Design review of the part built by this model. Coordinates are the model's own, in mm. Face numbers are marked on the shaded views. Round coordinates to 2 decimals unless told otherwise and drop trailing zeros. Write each loop counter-clockwise with the first axis right and the second up, starting at its lowest first coordinate (ties: lowest second). Pieces come first, ordered by that corner, then holes. Notation, with made-up numbers: (65.5, -26.75) - (89.5, -26.75) arc R21 ccw to (89.5, 2.25) - close; hole circle Ø2 at (-31, 34.5). An arc over 180 degrees is marked (long way). Use one line per item in the form item = value.
```python
from build123d import *

# Parameters (mm, degrees)
F0_W     = 50.6464093924
F0_H     = 100.5250141025
F1_DEPTH = 0.254
F0_W_2   = 58.674
F0_H_2   = 123.952
F2_DEPTH = 7.874
F3_R     = 9.8113639175
F4_R     = 9.8044
F6_W     = 12.2285038233
F6_H     = 3.6733425222
F7_DEPTH = 17.272
F8_R     = 2.2102361545
F9_DEPTH = 12.192


# Not quite as in the source:
# - the program builds the solid bodies; features that only make, move or delete a surface that nothing else refers to are left out


with BuildPart() as f1:
    # F0 (on Top) → F1 (new body)
    with BuildSketch(Plane.XY):
        with Locations((55.8215677738, 54.941402014)):
            Rectangle(F0_W, F0_H)
    extrude(amount=F1_DEPTH)

    # F0 (on Top) → F2 (join)
    with BuildSketch(Plane.XY):
        with Locations((55.8215677738, 54.941402014)):
            Rectangle(F0_W_2, F0_H_2)
        with Locations((55.8215677738, 54.941402014)):
            Rectangle(F0_W, F0_H, mode=Mode.SUBTRACT)
    extrude(amount=F2_DEPTH)

    # F3
    f3_edges = [f1.edges().sort_by_distance(p)[0] for p in [
        (26.484568, 116.917402, 3.937),
    ]]
    fillet(f3_edges, radius=F3_R)

    # F4
    f4_edges = [f1.edges().sort_by_distance(p)[0] for p in [
        (85.158568, 116.917402, 3.937),
    ]]
    fillet(f4_edges, radius=F4_R)

    # F6 (on face) → F7 (cut)
    with BuildSketch(Plane.XZ.offset(7.034597986)):
        with Locations((55.8215677738, 4.2473026551)):
            Rectangle(F6_W, F6_H)
    extrude(amount=-F7_DEPTH, mode=Mode.SUBTRACT)

    # F8 (on face) → F9 (cut)
    with BuildSketch(Plane.XZ.offset(7.034597986)):
        with Locations((35.0567772985, 3.8737377618)):
            Circle(F8_R)
    extrude(amount=-F9_DEPTH, mode=Mode.SUBTRACT)


solid = f1.part
```
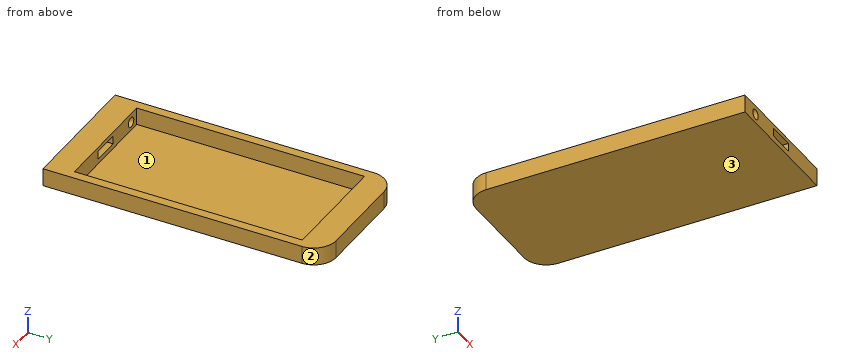
Q1. We need section D-D on x = 35. Write out the cut boundary in (y, z).
Calculated:
outline = (-7.03, 0) - (116.83, 0) - (116.83, 7.87) - (105.2, 7.87) - (105.2, 0.25) - (4.68, 0.25) - (4.68, 1.66) - (-7.03, 1.66) - close; (-7.03, 6.08) - (4.68, 6.08) - (4.68, 7.87) - (-7.03, 7.87) - close
Q2. We need section B-B on y = 6.5. Write out the cut boundary in (x, z).
Calculated:
outline = (26.48, 0) - (85.16, 0) - (85.16, 7.87) - (81.14, 7.87) - (81.14, 0.25) - (30.5, 0.25) - (30.5, 7.87) - (26.48, 7.87) - close
Q3. We need section A-A on x = 53.5. Write out the cut boundary in (y, z).
Calculated:
outline = (-7.03, 0) - (116.92, 0) - (116.92, 7.87) - (105.2, 7.87) - (105.2, 0.25) - (4.68, 0.25) - (4.68, 2.41) - (-7.03, 2.41) - close; (-7.03, 6.08) - (4.68, 6.08) - (4.68, 7.87) - (-7.03, 7.87) - close
Q4. To check wall thickness, follow line 1 along Y through (x, z) = (43, 7); line 2 along X through (y, z) = (61.5, 5.25); line 3 along Z through (x, y) = (61, 79). State the ranges of each line that lie inside material, in increasing order. Write a range as from..to.
Calculated:
line_1 = -7.03..4.68, 105.2..116.92
line_2 = 26.48..30.5, 81.14..85.16
line_3 = 0..0.25
Q5. For P1, Ø6, axis at x = 67, y = 75, coming from the +Z side, flat-tipped, find the tip position at first contact; note if it passes through.
Calculated:
P1 = 0.25
Q6. We need section C-C on x = 46. Write out the cut boundary in (y, z).
Calculated:
outline = (-7.03, 0) - (116.92, 0) - (116.92, 7.87) - (105.2, 7.87) - (105.2, 0.25) - (4.68, 0.25) - (4.68, 7.87) - (-7.03, 7.87) - close
Q7. Draft analysis for pull direction Y (two halves, no side actions). For the marked faces 1, 2 and 3, state which applies: released by +Y, released by -Y, zero draft, split by the parting line, or undercut.
Calculated:
face_1 = undercut
face_2 = released by +Y
face_3 = zero draft
